from build123d import *

# Parameters (mm, degrees)
SKETCH1_W                    = 271.78
SKETCH1_H                    = 156.21
BASE_FLANGE1_DEPTH           = 2.38125
EDGE_FLANGE1_STRIP_W         = 15.875
EDGE_FLANGE1_STRIP_H         = 2.38125
EDGE_FLANGE1_STRIP_CUT_DEPTH = 271.78
EDGE_FLANGE1_DEPTH           = 271.78
EDGE_FLANGE2_STRIP_W         = 15.875
EDGE_FLANGE2_STRIP_H         = 2.38125
EDGE_FLANGE2_STRIP_CUT_DEPTH = 153.035
EDGE_FLANGE2_DEPTH           = 153.035
SKETCH14_W                   = 127
SKETCH14_H                   = 30.097595223
CUT_EXTRUDE1_DEPTH           = 5.588
EDGE_FLANGE3_STRIP_W         = 15.875
EDGE_FLANGE3_STRIP_H         = 2.38125
EDGE_FLANGE3_STRIP_CUT_DEPTH = 153.035
EDGE_FLANGE3_DEPTH           = 153.035
SKETCH18_W                   = 127
SKETCH18_H                   = 45.504454023
CUT_EXTRUDE2_DEPTH           = 5.588
CUT_EXTRUDE3_START           = -3.302
CUT_EXTRUDE3_DEPTH           = 5.68325
CUT_EXTRUDE4_START           = -3.302
CUT_EXTRUDE4_DEPTH           = 5.68325
EDGE_FLANGE4_STRIP_W         = 15.875
EDGE_FLANGE4_STRIP_H         = 2.38125
EDGE_FLANGE4_STRIP_CUT_DEPTH = 265.3665
EDGE_FLANGE4_DEPTH           = 265.3665
SKETCH24_W                   = 190.754
SKETCH24_H                   = 70.532416994
CUT_EXTRUDE5_DEPTH           = 5.588
SKETCH25_W                   = 50.8
SKETCH25_H                   = 127
CUT_EXTRUDE6_DEPTH           = 2.54


# Read off the part's stored shape, not the designer's step: Cut-Extrude3, Cut-Extrude4
# Sheet-metal steps are written as plain solids
with BuildPart() as part:
    # Sketch1 → Base-Flange1 (new body)
    with BuildSketch(Plane(origin=(0, 0, 0), x_dir=(1, 0, 0), z_dir=(0, 1, 0))):
        Rectangle(SKETCH1_W, SKETCH1_H)
    extrude(amount=-BASE_FLANGE1_DEPTH)

    # Edge-Flange1 strip (across the edge) → Edge-Flange1 strip cut (cut)
    with BuildSketch(Plane(origin=(135.89, -2.38125, 78.105), x_dir=(0, 0, -1), z_dir=(-1, 0, 0))):
        with Locations((-4.7625, -1.190625)):
            Rectangle(EDGE_FLANGE1_STRIP_W, EDGE_FLANGE1_STRIP_H)
    extrude(amount=EDGE_FLANGE1_STRIP_CUT_DEPTH, mode=Mode.SUBTRACT)

    # Edge-Flange1 section (across the edge) → Edge-Flange1 (add)
    with BuildSketch(Plane(origin=(135.89, -2.38125, 78.105), x_dir=(0, 0, -1), z_dir=(-1, 0, 0))):
        with BuildLine():
            Line((-2.38125, 3.175), (-2.38125, 23.01875))
            Line((-2.38125, 23.01875), (0, 23.01875))
            Line((0, 23.01875), (0, 3.175))
            ThreePointArc((0, 3.175), (0.92993597, 0.92993597), (3.175, 0))
            Line((3.175, 0), (3.175, -2.38125))
            ThreePointArc((3.175, -2.38125), (-0.753862053, -0.753862053), (-2.38125, 3.175))
        make_face()
    extrude(amount=EDGE_FLANGE1_DEPTH)

    # Edge-Flange2 strip (across the edge) → Edge-Flange2 strip cut (cut)
    with BuildSketch(Plane(origin=(135.89, -2.38125, -78.105), x_dir=(-1, 0, 0), z_dir=(0, 0, 1))):
        with Locations((-4.7625, -1.190625)):
            Rectangle(EDGE_FLANGE2_STRIP_W, EDGE_FLANGE2_STRIP_H)
    extrude(amount=EDGE_FLANGE2_STRIP_CUT_DEPTH, mode=Mode.SUBTRACT)

    # Edge-Flange2 section (across the edge) → Edge-Flange2 (add)
    with BuildSketch(Plane(origin=(135.89, -2.38125, -78.105), x_dir=(-1, 0, 0), z_dir=(0, 0, 1))):
        with BuildLine():
            Line((-2.38125, 3.175), (-2.38125, 23.01875))
            Line((-2.38125, 23.01875), (0, 23.01875))
            Line((0, 23.01875), (0, 3.175))
            ThreePointArc((0, 3.175), (0.92993597, 0.92993597), (3.175, 0))
            Line((3.175, 0), (3.175, -2.38125))
            ThreePointArc((3.175, -2.38125), (-0.753862053, -0.753862053), (-2.38125, 3.175))
        make_face()
    extrude(amount=EDGE_FLANGE2_DEPTH)

    # Sketch14 → Cut-Extrude1 (cut)
    with BuildSketch(Plane(origin=(138.27125, 0, 0), x_dir=(0, 0, -1), z_dir=(1, 0, 0))):
        with Locations((14.605, -10.351202389)):
            Rectangle(SKETCH14_W, SKETCH14_H)
    extrude(amount=-CUT_EXTRUDE1_DEPTH, mode=Mode.SUBTRACT)

    # Edge-Flange3 strip (across the edge) → Edge-Flange3 strip cut (cut)
    with BuildSketch(Plane(origin=(-135.89, -2.38125, 74.93), x_dir=(1, 0, 0), z_dir=(0, 0, -1))):
        with Locations((-4.7625, -1.190625)):
            Rectangle(EDGE_FLANGE3_STRIP_W, EDGE_FLANGE3_STRIP_H)
    extrude(amount=EDGE_FLANGE3_STRIP_CUT_DEPTH, mode=Mode.SUBTRACT)

    # Edge-Flange3 section (across the edge) → Edge-Flange3 (add)
    with BuildSketch(Plane(origin=(-135.89, -2.38125, 74.93), x_dir=(1, 0, 0), z_dir=(0, 0, -1))):
        with BuildLine():
            Line((-2.38125, 3.175), (-2.38125, 23.01875))
            Line((-2.38125, 23.01875), (0, 23.01875))
            Line((0, 23.01875), (0, 3.175))
            ThreePointArc((0, 3.175), (0.92993597, 0.92993597), (3.175, 0))
            Line((3.175, 0), (3.175, -2.38125))
            ThreePointArc((3.175, -2.38125), (-0.753862053, -0.753862053), (-2.38125, 3.175))
        make_face()
    extrude(amount=EDGE_FLANGE3_DEPTH)

    # Sketch18 → Cut-Extrude2 (cut)
    with BuildSketch(Plane.ZY.offset(138.27125)):
        with Locations((-14.605, -2.647772988)):
            Rectangle(SKETCH18_W, SKETCH18_H)
    extrude(amount=-CUT_EXTRUDE2_DEPTH, mode=Mode.SUBTRACT)

    # Cut-Extrude3 outline → Cut-Extrude3 (cut)
    with BuildSketch(Plane.ZY.offset(135.89).offset(CUT_EXTRUDE3_START)):
        with BuildLine():
            Line((74.93, 0), (74.89825, 0))
            Line((74.89825, 0), (74.89825, -5.55625))
            Line((74.89825, -5.55625), (74.93, -5.55625))
            Line((74.93, -5.55625), (74.93, -2.38125))
            ThreePointArc((74.93, -2.38125), (77.17506403, -3.31118597), (78.105, -5.55625))
            Line((78.105, -5.55625), (78.105, -25.4))
            Line((78.105, -25.4), (80.48625, -25.4))
            Line((80.48625, -25.4), (80.48625, -5.55625))
            ThreePointArc((80.48625, -5.55625), (78.858862053, -1.627387947), (74.93, 0))
        make_face()
    extrude(amount=CUT_EXTRUDE3_DEPTH, mode=Mode.SUBTRACT)

    # Cut-Extrude4 outline → Cut-Extrude4 (cut)
    with BuildSketch(Plane(origin=(135.89, 0, 0), x_dir=(0, 0, -1), z_dir=(1, 0, 0)).offset(CUT_EXTRUDE4_START)):
        with BuildLine():
            Line((-74.89825, 0), (-74.93, 0))
            ThreePointArc((-74.93, 0), (-78.858862053, -1.627387947), (-80.48625, -5.55625))
            Line((-80.48625, -5.55625), (-80.48625, -25.4))
            Line((-80.48625, -25.4), (-78.105, -25.4))
            Line((-78.105, -25.4), (-78.105, -5.55625))
            ThreePointArc((-78.105, -5.55625), (-77.17506403, -3.31118597), (-74.93, -2.38125))
            Line((-74.93, -2.38125), (-74.93, -5.55625))
            Line((-74.93, -5.55625), (-74.89825, -5.55625))
            Line((-74.89825, -5.55625), (-74.89825, 0))
        make_face()
    extrude(amount=CUT_EXTRUDE4_DEPTH, mode=Mode.SUBTRACT)

    # Edge-Flange4 strip (across the edge) → Edge-Flange4 strip cut (cut)
    with BuildSketch(Plane(origin=(-132.68325, -2.38125, -78.105), x_dir=(0, 0, 1), z_dir=(1, 0, 0))):
        with Locations((-4.7625, -1.190625)):
            Rectangle(EDGE_FLANGE4_STRIP_W, EDGE_FLANGE4_STRIP_H)
    extrude(amount=EDGE_FLANGE4_STRIP_CUT_DEPTH, mode=Mode.SUBTRACT)

    # Edge-Flange4 section (across the edge) → Edge-Flange4 (add)
    with BuildSketch(Plane(origin=(-132.68325, -2.38125, -78.105), x_dir=(0, 0, 1), z_dir=(1, 0, 0))):
        with BuildLine():
            Line((-2.38125, 3.175), (-2.38125, 23.01875))
            Line((-2.38125, 23.01875), (0, 23.01875))
            Line((0, 23.01875), (0, 3.175))
            ThreePointArc((0, 3.175), (0.92993597, 0.92993597), (3.175, 0))
            Line((3.175, 0), (3.175, -2.38125))
            ThreePointArc((3.175, -2.38125), (-0.753862053, -0.753862053), (-2.38125, 3.175))
        make_face()
    extrude(amount=EDGE_FLANGE4_DEPTH)

    # Sketch24 → Cut-Extrude5 (cut)
    with BuildSketch(Plane.XY.offset(80.48625)):
        Rectangle(SKETCH24_W, SKETCH24_H)
    extrude(amount=-CUT_EXTRUDE5_DEPTH, mode=Mode.SUBTRACT)

    # Sketch25 → Cut-Extrude6 (cut)
    with BuildSketch(Plane(origin=(0, 0, 0), x_dir=(1, 0, 0), z_dir=(0, 1, 0))):
        Rectangle(SKETCH25_W, SKETCH25_H)
    extrude(amount=-CUT_EXTRUDE6_DEPTH, mode=Mode.SUBTRACT)


solid = part.part
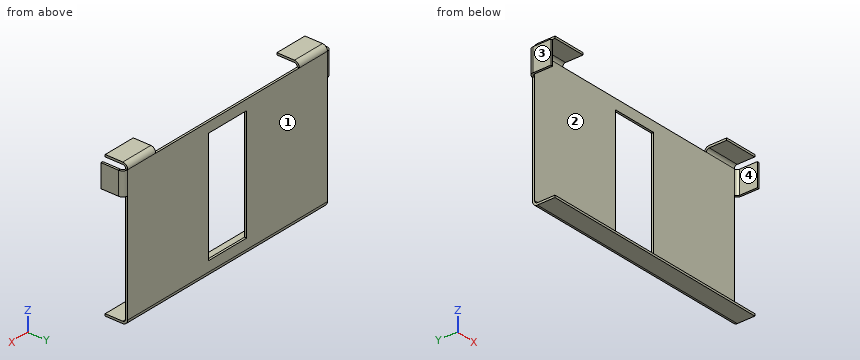
Can you work these out from the model? Positions are in its coordinate system, mm. Face numbers are marked on the shaded views. Give positions to 0.01 mm unless a question says otherwise; leave off trailing zeros. Write each loop counter-clockwise with the first axis right and the second up, starting at its lowest first coordinate (ties: lowest second). Pieces come first, ordered by that corner, then holes. Notation, with made-up numbers: M 48,22.25 L 97,22.25 A17 cw 97,45.25 Z; hole C 32,53 d7. An arc over 180 degrees is marked long. Answer in a Markdown table with one row per item. Add a question column.
Item 1: Imagine slicing it at C-C, the plane y = -19.75. Write out the boundary of the cut face in (x, z) (3 decimals), plus the area to 3 significant figures.
Item 2: We'd pull the mould along X, two halves only. Please class the marked faces 1, 2, 3 and 4: released by +X, released by -X, zero draft, split by the parting line, or undercut.
Item 3: Please list where these lines run through material, in increasing order: L1, parallel to X at y = -23.75, z = 50.5; L2, parallel to X at y = -1.5, z = -62; L3, parallel to Y at x = -80, z = 42.5.
Item 4: For pin 1 Ø10 at (y, z) = (-4.5, -41.5) entering from -X; pin 2 Ø1.7 at (x, y) = (135, -15.5) entering from -Z; pin 3 Ø1.7 at (y, z) = (-7.5, 77.5) entering from -X; pin 4 Ø4 at (x, y) = (89, -4) entering from +Z, each with a flat end and sliding along its axis, tell me the tip position at first contact or that it passes through.
Item 5: Imagine slicing it at A-A, the plane z = -8.5. Write out the boundary of the cut face in (x, y), plus the area to 3 significant figures.
Evaluation:
| question | item | result |
|---|---|---|
| 1 | outline | M -138.271,48.895 L -135.89,48.895 L -135.89,74.93 L -138.271,74.93 Z; M -132.683,-80.486 L 132.683,-80.486 L 132.683,-78.105 L -132.683,-78.105 Z; M -132.588,78.105 L -95.377,78.105 L -95.377,80.486 L -132.588,80.486 Z; M 95.377,78.105 L 132.588,78.105 L 132.588,80.486 L 95.377,80.486 Z; M 135.89,48.895 L 138.271,48.895 L 138.271,74.93 L 135.89,74.93 Z |
| 1 | area | 933 mm² |
| 2 | face 1 | zero draft |
| 2 | face 2 | undercut |
| 2 | face 3 | released by -X |
| 2 | face 4 | undercut |
| 3 | L1 | x = -138.27 to -135.89, 135.89 to 138.27 |
| 3 | L2 | x = -132.68 to -25.4, 25.4 to 132.68 |
| 3 | L3 | y = -2.38 to 0 |
| 4 | pin 1 | stops at x = -132.68 |
| 4 | pin 2 | passes through |
| 4 | pin 3 | stops at x = -132.59 |
| 4 | pin 4 | stops at z = 74.9 |
| 5 | outline | M -132.68,-2.38 L -25.4,-2.38 L -25.4,0 L -132.68,0 Z; M 25.4,-2.38 L 132.68,-2.38 L 132.68,0 L 25.4,0 Z |
| 5 | area | 511 mm² |
